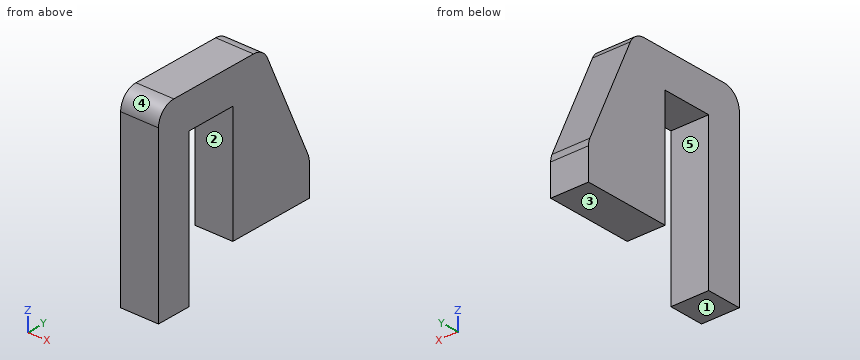
Autodesk Inventor part; units mm, degrees
ref_plane "YZ Plane" through (0, 0, 0) normal (1, 0, 0) x (0, 1, 0)
ref_plane "XZ Plane" through (0, 0, 0) normal (0, 1, 0) x (-1, 0, 0)
ref_plane "XY Plane" through (0, 0, 0) normal (0, 0, 1) x (1, 0, 0)
sketch "Sketch1" plane through (0, 0, 0) normal (1, 0, 0) x (0, 1, 0)
  line L0 (0, 0) -> (0, 21.3)
  line L1 (0, 21.3) -> (13.7, 21.3)
  line L2 (19.7, 4) -> (9.7, 4)
  line L3 (9.7, 4) -> (9.7, 17.3)
  line L4 (9.7, 17.3) -> (4, 17.3)
  line L5 (4, 17.3) -> (4, 0)
  line L6 (4, 0) -> (0, 0)
  line L7 (13.7, 21.3) -> (19.7, 8)
  line L8 (19.7, 8) -> (19.7, 4)
  dimension "d0" = 4
  dimension "d1" = 4
  dimension "d2" = 5.7
  dimension "d4" = 4
  dimension "d5" = 10
  dimension "d6" = 13.3
  dimension "d9" = 4
  dimension "d11" = 4
extrude "Extrusion1" add sketch "Sketch1" along normal blind 4.3
fillet "Fillet1" radius 2 3 edges at (2.15, 0, 21.3) (2.15, 13.7, 21.3) (2.15, 19.7, 8)
properties part number "TrayPanelJ"
Input: part model. Units: mm. Frame: model coordinates. Face numbers are marked on the shaded views. A direction names the side the tool comes from. Give positions to 0.01 mm unless a question says otherwise; leave off trailing zeros. Order: outer loops, then holes, each group sorted by start corner. A loop starts at its lowest first (then second) coordinate and runs counter-clockwise, first axis right, second up. Notation, with made-up numbers: (53, -32) - (89, -32) arc R36 ccw to (89, 3) - close; hole circle Ø8 at (37.5, -13.75). An arc over 180 degrees is marked (long way). Answer as a JSON object with one key per item and string values. Group by question number.
Q1. Cut plane D-D, the plane z = 7.25. Output: boundary loops of the cut face in (x, y), then the cut area to 3 significant figures.
Q2. Cut plane C-C, the plane y = 11.5. Output: boundary loops of the cut face in (x, z).
Q3. Cut plane B-B, the plane x = 1.2. Output: boundary loops of the cut face in (y, z), then the cut area to 3 significant figures.
Q4. Cut plane A-A, the plane z = 14.25. Output: boundary loops of the cut face in (x, y).
Q5. Mould query, pull axis Y, two halves, no side actions, for the marked faces 3, 4 and 5. Classes: pulls with the +Y half, pulls with the -Y half, needs draft (parallel to the pull), parting line crosses it, or undercut.
Q6. Set-up query: the marked faces 1 and 2. Return all of +Z, -Z, +X, -X, +Y, -Y with unobstructed straight access to the full face (end or side cutting, diameter ignored); none if empty.
Q7. Line query: probe 1 along Y at (x, z) = (3.1, 4.5); probe 2 along Z at (x, y) = (3.8, 8); probe 3 along Y at (x, z) = (2.55, 14). Output: solid intervals per line, ascending.
Q8. First-contact query: pin 1 Ø1.5 at (x, y) = (2, 16.5) entering from +Z; pin 2 Ø1.3 at (x, y) = (1, 14.5) entering from -Z; pin 3 Ø2 at (x, z) = (3, 11.5) entering from -Y; pin 4 Ø2 at (x, z) = (1.5, 10) entering from +Y. Flat tips, straight axial feed; report the tip coordinate or a pass-through.
Results:
{
 "1": {"outline": "(0, 0) - (4.3, 0) - (4.3, 4) - (0, 4) - close; (0, 9.7) - (4.3, 9.7) - (4.3, 19.7) - (0, 19.7) - close", "area": "60.2 mm^2"},
 "2": {"outline": "(0, 4) - (4.3, 4) - (4.3, 21.3) - (0, 21.3) - close"},
 "3": {"outline": "(0, 0) - (4, 0) - (4, 17.3) - (9.7, 17.3) - (9.7, 4) - (19.7, 4) - (19.7, 7.57) arc R2 ccw to (19.52, 8.39) - (14.23, 20.12) arc R2 ccw to (12.41, 21.3) - (2, 21.3) arc R2 ccw to (0, 19.3) - close", "area": "240 mm^2"},
 "4": {"outline": "(0, 0) - (4.3, 0) - (4.3, 4) - (0, 4) - close; (0, 9.7) - (4.3, 9.7) - (4.3, 16.88) - (0, 16.88) - close"},
 "5": {"face 3": "needs draft", "face 4": "pulls with the -Y half", "face 5": "undercut"},
 "6": {"face 1": "-Z, +X, -X, +Y, -Y", "face 2": "-Z, +X, -X"},
 "7": {"probe 1": "0 to 4, 9.7 to 19.7", "probe 2": "17.3 to 21.3", "probe 3": "0 to 4, 9.7 to 16.99"},
 "8": {"pin 1": "z = 16.76", "pin 2": "z = 4", "pin 3": "y = 0", "pin 4": "y = 19.25"}
}
